Could you check a few things on this drawing? It's one solid part, dimensions in mm from its lowest x, y, z. A direction names the side the tool comes from. Give positions to 0.01 mm unless a question says otherwise; leave off trailing zeros. Order: outer loops, then holes, each group sorted by start corner. A loop starts at its lowest first (then second) coordinate and runs counter-clockwise, first axis right, second up. Notation, with made-up numbers: M 29.25,56 L 43.25,56 A22 cw 43.25,67 Z; hole C 74.25,34 d3. An arc over 180 degrees is marked long. Use one line per item in the form item = value. Start each with the question number.
1. I need wall thicknesses on L1, parallel to Y at x = 8, z = 1.75; L2, parallel to Y at x = 15, z = 9.25; L3, parallel to Z at x = 5.75, y = 14.75. Which ranges of each line are inside material? Lowest first, please.
2. We'd pull the mould along Y, two halves only. Please class the marked faces 1, 2 and 3: +Y half, -Y half, draft (parallel to the pull), parting line (faces both ways), or undercut.
3. I want a section at C-C, the plane y = 4.25. List the corners of the cut face in (x, z) for me.
4. I want a section at D-D, the plane z = 4.75. List the corners of the cut face in (x, y) for me.
5. I want a section at B-B, the plane x = 8. List the corners of the cut face in (y, z) for me.
6. I want a section at A-A, the plane z = 8. List the corners of the cut face in (x, y) for me.
7. Will these pins go through, and if not, where does the flat tip stop? P1, Ø5, axis at y = 3.5, z = 2.5, coming from the +X side; P2, Ø6, axis at y = 9.5, z = 14.5, coming from the +X side; P3, Ø3, axis at x = 8, z = 8, coming from the -Y side; P4, Ø1, axis at x = 3, y = 2, coming from the +Z side.
8. For the marked faces 4, 5 and 6, which set-ups out of +Z, -Z, +X, -X, +Y, -Y let a thin tool reach every point of the face, with its end or its side?
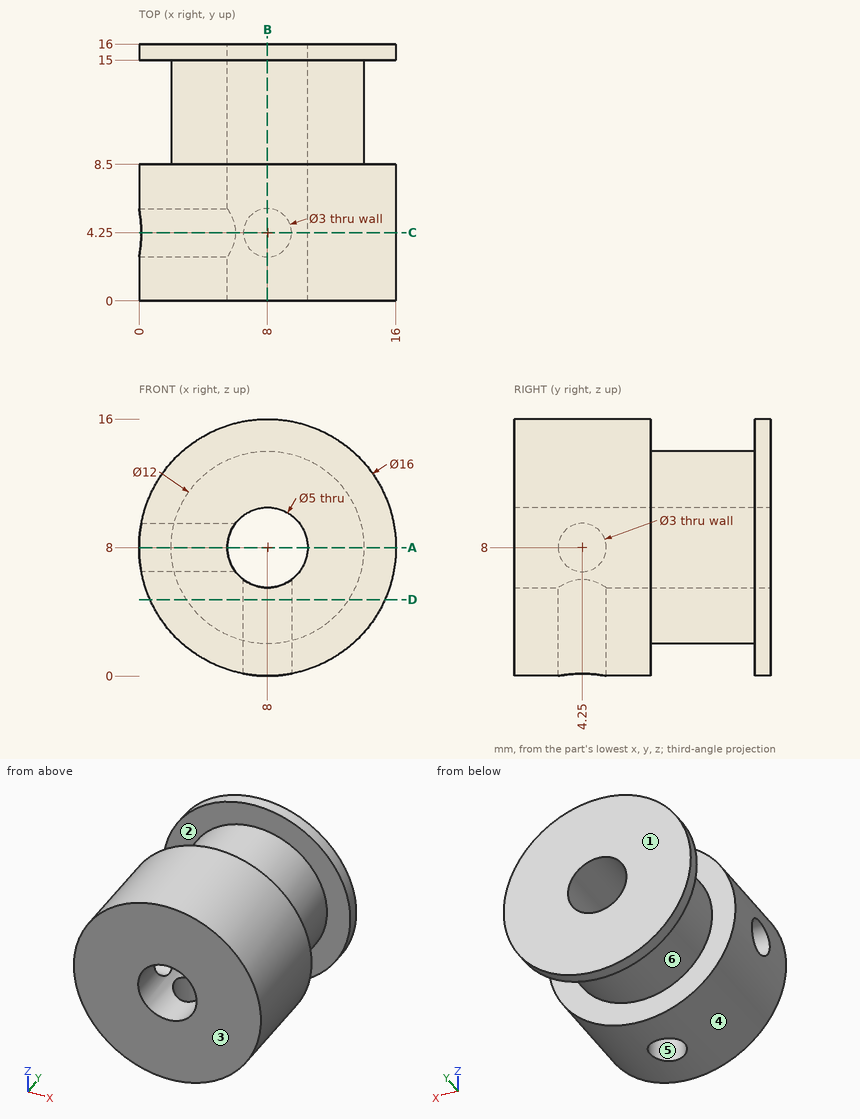
Check result:
q1.L1 = 0 to 2.75, 5.75 to 8.5, 15 to 16
q1.L2 = 0 to 8.5, 15 to 16
q1.L3 = 2.44 to 6.91, 9.09 to 13.56
q2.face_1 = +Y half
q2.face_2 = undercut
q2.face_3 = -Y half
q3.outline = M 0.14,6.5 A8 ccw 6.5,0.14 L 6.5,6 A2.5 cw 6,6.5 Z; M 0.14,9.5 L 6,9.5 A2.5 cw long 9.5,6 L 9.5,0.14 A8 ccw long Z
q4.outline = M 0.69,0 L 15.31,0 L 15.31,8.5 L 13.04,8.5 L 13.04,15 L 15.31,15 L 15.31,16 L 0.69,16 L 0.69,15 L 2.96,15 L 2.96,8.5 L 0.69,8.5 Z; hole C 8,4.25 d3
q5.outline = M 0,0 L 2.75,0 L 2.75,5.5 L 0,5.5 Z; M 0,10.5 L 16,10.5 L 16,16 L 15,16 L 15,14 L 8.5,14 L 8.5,16 L 0,16 Z; M 5.75,0 L 8.5,0 L 8.5,2 L 15,2 L 15,0 L 16,0 L 16,5.5 L 5.75,5.5 Z
q6.outline = M 0,0 L 5.5,0 L 5.5,2.75 L 0,2.75 Z; M 0,5.75 L 5.5,5.75 L 5.5,16 L 0,16 L 0,15 L 2,15 L 2,8.5 L 0,8.5 Z; M 10.5,0 L 16,0 L 16,8.5 L 14,8.5 L 14,15 L 16,15 L 16,16 L 10.5,16 Z
q7.P1 = 15.42
q7.P2 = 15.11
q7.P3 = through
q7.P4 = 14.61
q8.face_4 = +Y, -Y
q8.face_5 = -Z
q8.face_6 = none
